Here's how the part is built. I have some questions about the finished solid (model axes, mm). Face numbers are marked on the shaded views. A direction names the side the tool comes from. Round coordinates to 2 decimals unless told otherwise and drop trailing zeros. Loops run counter-clockwise (first coordinate to the right, second up) from the corner with the lowest first, then second, coordinate; pieces in that order, holes last. Notation, with made-up numbers: M -4.75,16 L 39.25,16 A28 ccw 39.25,51 Z; hole C -0.5,-38 d7. An arc over 180 degrees is marked long. Answer as a JSON object with one key per item and string values.
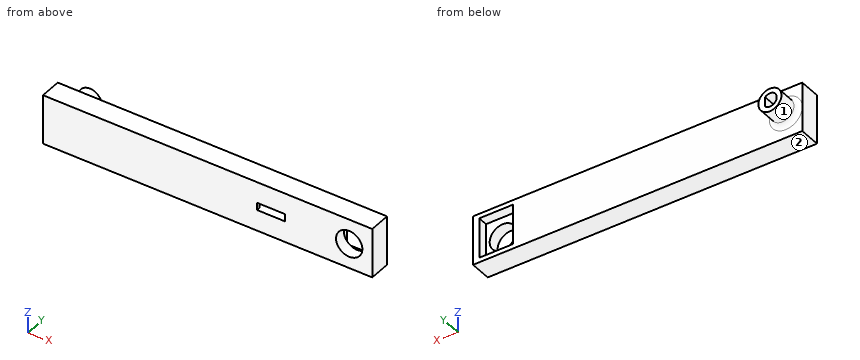
from build123d import *

# Parameters (mm, degrees)
SKETCH2_W                = 100
SKETCH2_H                = 15
BOSS_EXTRUDE1_DEPTH      = 3.25
SKETCH15_W               = 8.5
SKETCH15_H               = 4.25
SKETCH15_W_2             = 5
SKETCH15_H_2             = 3.25
CUT_EXTRUDE8_DEPTH       = 1.125
SKETCH18_W               = 10.2
SKETCH18_H               = 12.2
CUT_EXTRUDE10_DEPTH      = 3
CUT_EXTRUDE11_DEPTH      = 51.975484304
CUT_EXTRUDE11_DEPTH_BACK = 51.975484304
SKETCH19_R               = 4
SKETCH20_R               = 3.5
BOSS_EXTRUDE2_DEPTH      = 7
CUT_EXTRUDE12_DEPTH      = 9.5
FILLET1_R                = 1.5


with BuildPart() as part:
    # Sketch2 → Boss-Extrude1 (new, symmetric)
    with BuildSketch(Plane(origin=(0, 0, 0), x_dir=(1, 0, 0), z_dir=(0, 1, 0))):
        Rectangle(SKETCH2_W, SKETCH2_H)
    extrude(amount=BOSS_EXTRUDE1_DEPTH, both=True)

    # Sketch15 → Cut-Extrude8 (cut, symmetric)
    with BuildSketch(Plane.XY):
        with Locations((19.25, -1.125)):
            Rectangle(SKETCH15_W, SKETCH15_H)
        with Locations((12.5, -0.625)):
            Rectangle(SKETCH15_W_2, SKETCH15_H_2)
    extrude(amount=CUT_EXTRUDE8_DEPTH, both=True, mode=Mode.SUBTRACT)

    # Sketch18 → Cut-Extrude10 (cut)
    with BuildSketch(Plane(origin=(0, 3.25, 0), x_dir=(1, 0, 0), z_dir=(0, 1, 0))):
        with Locations((43, 0)):
            Rectangle(SKETCH18_W, SKETCH18_H)
    extrude(amount=-CUT_EXTRUDE10_DEPTH, mode=Mode.SUBTRACT)

    # Sketch19 → Cut-Extrude11 (cut, two sides: drawn at the far end of the back side and taken through both)
    with BuildSketch(Plane.XZ.offset(3.25).offset(-CUT_EXTRUDE11_DEPTH_BACK)):
        with Locations(Location((43, 0, 0), (0, 0, 270))):
            Circle(SKETCH19_R)
    extrude(amount=CUT_EXTRUDE11_DEPTH + CUT_EXTRUDE11_DEPTH_BACK, mode=Mode.SUBTRACT)

    # Sketch20 → Boss-Extrude2 (add)
    with BuildSketch(Plane(origin=(0, 3.25, 0), x_dir=(1, 0, 0), z_dir=(0, 1, 0))):
        with Locations(Location((-45, 0, 0), (0, 0, 90))):
            Circle(SKETCH20_R)
    extrude(amount=BOSS_EXTRUDE2_DEPTH)

    # Sketch21 → Cut-Extrude12 (cut)
    with BuildSketch(Plane(origin=(0, 10.25, 0), x_dir=(1, 0, 0), z_dir=(0, 1, 0))):
        with BuildLine():
            Line((-43.525, -1.459451952), (-43.525, 1.459451952))
            ThreePointArc((-43.525, 1.459451952), (-47.075, 0), (-43.525, -1.459451952))
        make_face()
    extrude(amount=-CUT_EXTRUDE12_DEPTH, mode=Mode.SUBTRACT)

    # Fillet1
    fillet1_edges = [part.edges().sort_by_distance(p)[0] for p in [
        (-45, 3.25, 3.5),
    ]]
    fillet(fillet1_edges, radius=FILLET1_R - 0.0001)  # a hair under: the kernel refuses the full size


solid = part.part
Item 1: For the marked faces 1 and 2, which set-ups out of +Z, -Z, +X, -X, +Y, -Y let a thin tool reach every point of the face, with its end or its side?
Solution:
{"face 1": "+Y", "face 2": "-Z, +X, -X, +Y, -Y"}
Item 2: I want a section at D-D on x = -45. List the corners of the cut face in (y, z) for me (3 decimals), plus the area to 3 significant figures.
Solution:
{"outline": "M -3.25,-7.5 L 3.25,-7.5 L 3.25,-5 A1.5 cw 4.75,-3.5 L 10.25,-3.5 L 10.25,-2.075 L 0.75,-2.075 L 0.75,2.075 L 10.25,2.075 L 10.25,3.5 L 4.75,3.5 A1.5 cw 3.25,5 L 3.25,7.5 L -3.25,7.5 Z", "area": "108 mm2"}
Item 3: I want a section at B-B on x = 43. List the corners of the cut face in (y, z) for me.
Solution:
{"outline": "M -3.25,-7.5 L 3.25,-7.5 L 3.25,-6.1 L 0.25,-6.1 L 0.25,-4 L -3.25,-4 Z; M -3.25,4 L 0.25,4 L 0.25,6.1 L 3.25,6.1 L 3.25,7.5 L -3.25,7.5 Z"}
Item 4: For P1, Ø2.5, axis at x = 11.5, z = 0, coming from the +Y side; P2, Ø1.1, axis at x = -45.5, z = 0.5, coming from the +Y side; P3, Ø1.5, axis at y = 6.5, z = 0.5, coming from the -X side, each with a flat end and sliding along its axis, tell me the tip position at first contact or that it passes through.
Solution:
{"P1": "stops at y = 3.25", "P2": "stops at y = 0.75", "P3": "stops at x = -48.5"}
Item 5: If I drill on L1, parallel to X at y = -1.55, z = 0; L2, parallel to X at y = 2, z = -0.25 (3 decimals); L3, parallel to X at y = 2, z = -5, over which ranges is the centre line in solid material (lowest first)? Write a range as from..to.
Solution:
{"L1": "x = -50..10, 23.5..39, 47..50", "L2": "x = -50..-47.06, -43.525..37.9, 48.1..50", "L3": "x = -50..37.9, 48.1..50"}
Item 6: I want a section at C-C on y = 8. List the corners of the cut face in (x, z) for me (3 decimals), plus the area to 3 significant figures.
Solution:
{"outline": "C -45,0 d7; hole M -43.525,-1.459 L -43.525,1.459 A2.075 ccw long Z", "area": "26.2 mm2"}
